Check sheet for the modelled part. Datum: model origin and axes. Units: mm. A direction names the side the tool comes from. Give positions to 0.01 mm unless a question says otherwise; leave off trailing zeros. Order: outer loops, then holes, each group sorted by start corner. A loop starts at its lowest first (then second) coordinate and runs counter-clockwise, first axis right, second up. Notation, with made-up numbers: M 67,87 L 113,87 A17 cw 113,111 Z; hole C 37,41 d3. An arc over 180 degrees is marked long. One line per question, with ' | ' between items. Start each with the question number.
Autodesk Inventor part; units mm, degrees
ref_plane "YZ Plane" through (0, 0, 0) normal (1, 0, 0) x (0, 1, 0)
ref_plane "XZ Plane" through (0, 0, 0) normal (0, 1, 0) x (-1, 0, 0)
ref_plane "XY Plane" through (0, 0, 0) normal (0, 0, 1) x (1, 0, 0)
sketch "Sketch1" plane through (0, 0, 0) normal (0, 0, 1) x (1, 0, 0)
  circle A0 centre (0, 0) radius 2
  dimension "d0" = 4
extrude "Extrusion1" add sketch "Sketch1" along normal blind 47
sketch "Sketch2" plane through (0, 0, 47) normal (0, 0, 1) x (1, 0, 0)
  circle A0 centre (0, 0) radius 2
  circle A1 centre (0, 0) radius 3
  dimension "d3" = 6
extrude "Extrusion2" add sketch "Sketch2" along normal blind 5
extrude "Extrusion3" add sketch "Sketch2" along normal blind 2 contours A0
sketch "Sketch3" plane through (0, 0, 0) normal (0, 0, -1) x (-1, 0, 0)
  circle A0 centre (0, 0) radius 3
extrude "Extrusion4" add sketch "Sketch3" along normal blind 5
sketch "Sketch4" plane through (0, 0, -5) normal (0, 0, -1) x (-1, 0, 0)
  circle A0 centre (0, 0) radius 2
  dimension "d10" = 4
extrude "Extrusion5" cut sketch "Sketch4" against normal blind 3
properties part number "Fake Bolt" material "Steel"
Item 1: Set-up check for faces 1 (the face through (0, -2, -4)), 2 (the face through (1, -2, 52)), 3 (the face through (0, 2, 50)), 4 (the face through (3, 0, -2)), 5 (the face through (-1, -2, 0)): record each of +Z, -Z, +X, -X, +Y, -Y from which the full face is reachable in a straight line by a thin tool's end or side.
Item 2: Section check C-C, the plane z = 6. Record the cut outline in (x, y).
Item 3: Section check A-A, the plane x = 0. Record the cut outline in (y, z).
Item 4: Draft check along X on faces 6 (the face through (-1, -2, -5)), 7 (the face through (-3, 0, 49)), 8 (the face through (0, 0, 49)). Enter one of: released by +X, released by -X, zero draft, split by the parting line, or undercut.
Item 5: Scan lines: probe 1 along Z at (x, y) = (0.9, -2.45); probe 2 along Y at (x, z) = (0, -4); probe 3 along Z at (x, y) = (-1.7, -0.75). Record each from-to range of solid material in increasing order. Write a range as [from, to].
Item 6: Go/stop test with flat-tipped pins: P1, Ø1.2, axis at x = 0.5, y = 0.5, coming from the -Z side; P2, Ø3.5, axis at x = 0, y = 0, coming from the +Z side. Record where each tip stops, or that it passes through.
Reported:
1) face 1: -Z | face 2: +Z, +X, -X, +Y, -Y | face 3: +Z | face 4: +Z, -Z | face 5: none
2) outline: C 0,0 d4
3) outline: M -3,-5 L -2,-5 L -2,-2 L 2,-2 L 2,-5 L 3,-5 L 3,0 L 2,0 L 2,47 L 3,47 L 3,52 L 2,52 L 2,49 L -2,49 L -2,52 L -3,52 L -3,47 L -2,47 L -2,0 L -3,0 Z
4) face 6: zero draft | face 7: split by the parting line | face 8: undercut
5) probe 1: z = [-5, 0], [47, 52] | probe 2: y = [-3, -2], [2, 3] | probe 3: z = [-2, 49]
6) P1: stops at z = -2 | P2: stops at z = 49
